```python
from build123d import *

# Parameters (mm, degrees)
F2_R = 5


with BuildPart() as f1:
    # F0 (on Right) → F1 (revolve)
    with BuildSketch(Plane.YZ):
        with BuildLine():
            Line((8, -38.566649), (12.832926, -38.566649))
            Line((12.832926, -38.566649), (12.996954, -38.392151))
            Line((12.996954, -38.392151), (12.850376, -34.19471))
            ThreePointArc((12.850376, -34.19471), (11.566748, -30.726), (9.06815, -27.998977))
            Line((9.06815, -27.998977), (7.319139, -1.46226))
            ThreePointArc((7.319139, -1.46226), (6.953716, -0.434518), (5.953226, 0))
            Line((5.953226, 0), (0, 0))
            Line((0, 0), (0, -8.266649))
            Line((0, -8.266649), (3.55, -8.266649))
            Line((3.55, -8.266649), (5, -30.266649))
            ThreePointArc((5, -30.266649), (7.030814, -31.89776), (7.853422, -34.369207))
            Line((7.853422, -34.369207), (8, -38.566649))
        make_face()
    revolve(axis=Axis((0, 0, -4.133324), (0, 0, 1)))

    # F2
    f2_edges = [f1.edges().sort_by_distance(p)[0] for p in [
        (0, -9.06815, -27.998977),
    ]]
    fillet(f2_edges, radius=F2_R)


solid = f1.part
```
Input: part model. Units: mm. Frame: model coordinates. Round coordinates to 2 decimals unless told otherwise and drop trailing zeros. Write each loop counter-clockwise with the first axis right and the second up, starting at its lowest first coordinate (ties: lowest second). Pieces come first, ordered by that corner, then holes. Notation, with made-up numbers: (22.25, 55) -> (35.25, 55) arc R20 cw to (35.25, 93) -> close; hole circle Ø9 at (-12, -10.75). An arc over 180 degrees is marked (long way). Answer as CSV lines item,"result".
1. Section B-B (z = -4). Return the cut outline in (x, y).
Geometry says:
outline,"circle Ø14.97 at (0, 0)"
2. Mould query, pull axis X, two halves, no side actions, for faces 1 (the conical face through (12.6, -2.8, -35.8)), 2 (the flat face through (0, 0, -8.267)), 3 (the flat face through (6, 6, -38.567)). Classes: +X half, -X half, draft (parallel to the pull), parting line (faces both ways), or undercut.
Geometry says:
face 1,"parting line"
face 2,"undercut"
face 3,"draft"
3. Contact query for flat-ended pins moving along their axis: P1, Ø1, axis at x = 10, y = 9, coming from the -Z side; P2, Ø1.5, axis at y = 2.5, z = -5, coming from the -X side; P3, Ø8, axis at y = 9, z = -22, coming from the +X side. Output: stop coordinate, or through.
Geometry says:
P1,"stops at z = -38.44"
P2,"stops at x = -7.35"
P3,"stops at x = 7.1"
4. Ray query, L1, parallel to Z at x = 1, y = -0.25; L2, parallel to Y at x = 0, z = -12; L3, parallel to Y at x = -1.5, z = -11. Return the intervals inside material, ascending. Write a range as [from, to].
Geometry says:
L1,"z = [-8.27, 0]"
L2,"y = [-8.01, -3.8], [3.8, 8.01]"
L3,"y = [-7.8, -3.42], [3.42, 7.8]"
5. Section C-C (z = -23). Return the cut outline in (x, y), plus the area to 3 significant figures.
Geometry says:
outline,"circle Ø17.48 at (0, 0); hole circle Ø9.04 at (0, 0)"
area,"176 mm^2"
6. Section A-A (z = -36). Return the cut outline in (x, y).
Geometry says:
outline,"circle Ø25.83 at (0, 0); hole circle Ø15.82 at (0, 0)"
